Drawing for the job (mm, zero at the part's lowest x, y, z). Coordinates: 2 decimals unless noted, no trailing zeros. Order: outer loops, then holes, each group sorted by start corner. A loop starts at its lowest first (then second) coordinate and runs counter-clockwise, first axis right, second up.
1) Cut at B-B (x = 61.5). List the corners of the cut face in (y, z), and give its area (3 significant figures).
2) Cut at A-A (z = 15). List the corners of the cut face in (x, y) (3 decimals), and give its area (3 significant figures).
3) Cut at C-C (y = 3.35). List the corners of the cut face in (x, z) (3 decimals).
4) Wall check: L1, parallel to X at y = 3.15, z = 7.5; L2, parallel to X at y = 2.8, z = 18.5; L3, parallel to Y at x = 34.5, z = 1.75. Give the ranges that are in metal, low to high.
5) Mould opens along Y. For the marked faces 1 and 2 say: +Y half, -Y half, draft (parallel to the pull), parting line (faces both ways), or undercut.
6) Cut at D-D (x = 11.5). List the corners of the cut face in (y, z) (3 decimals).
7) Pin check, flat tip, straight feed: pin 1 Ø2 at (x, z) = (61, 4) entering from +Y. Stop position of the tip, or through.
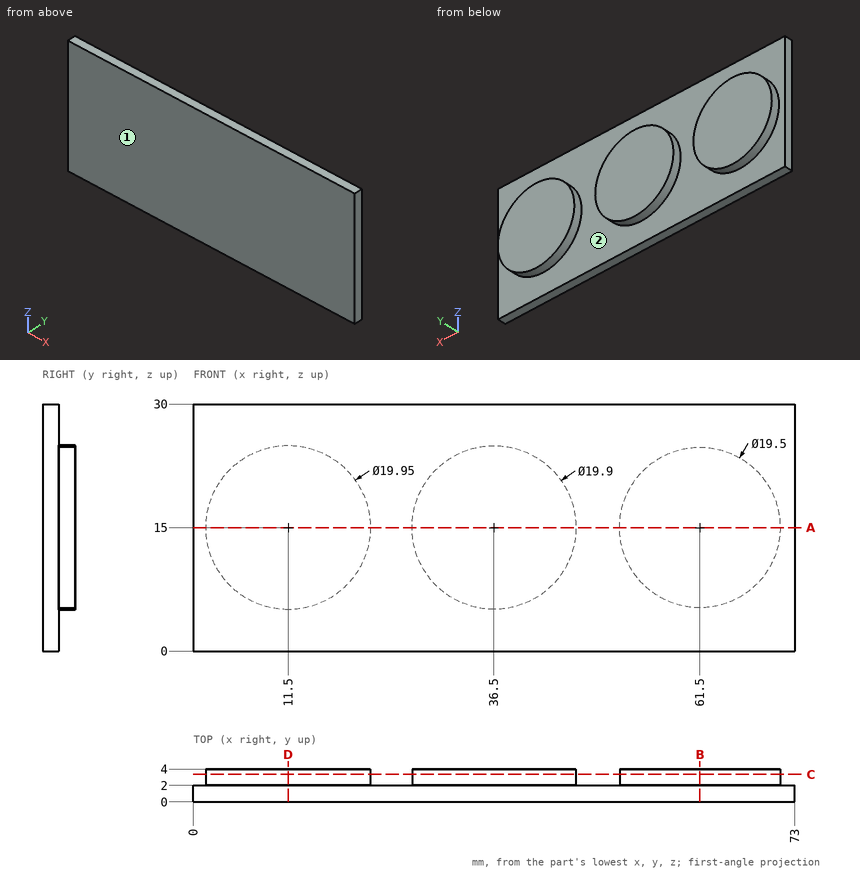
Geometry check:
1. outline: (0, 0) - (2, 0) - (2, 5.25) - (4, 5.25) - (4, 24.75) - (2, 24.75) - (2, 30) - (0, 30) - close
1. area: 99.0 mm2
2. outline: (0, 0) - (73, 0) - (73, 2) - (71.25, 2) - (71.25, 4) - (51.75, 4) - (51.75, 2) - (46.45, 2) - (46.45, 4) - (26.55, 4) - (26.55, 2) - (21.475, 2) - (21.475, 4) - (1.525, 4) - (1.525, 2) - (0, 2) - close
2. area: 265 mm2
3. outline: circle Ø19.95 at (11.5, 15); circle Ø19.9 at (36.5, 15); circle Ø19.5 at (61.5, 15)
4. L1: x = 4.92 to 18.08, 29.96 to 43.04, 55.27 to 67.73
4. L2: x = 2.16 to 20.84, 27.19 to 45.81, 52.4 to 70.6
4. L3: y = 0 to 2
5. face 1: -Y half
5. face 2: +Y half
6. outline: (0, 0) - (2, 0) - (2, 5.025) - (4, 5.025) - (4, 24.975) - (2, 24.975) - (2, 30) - (0, 30) - close
7. pin 1: stops at y = 2
